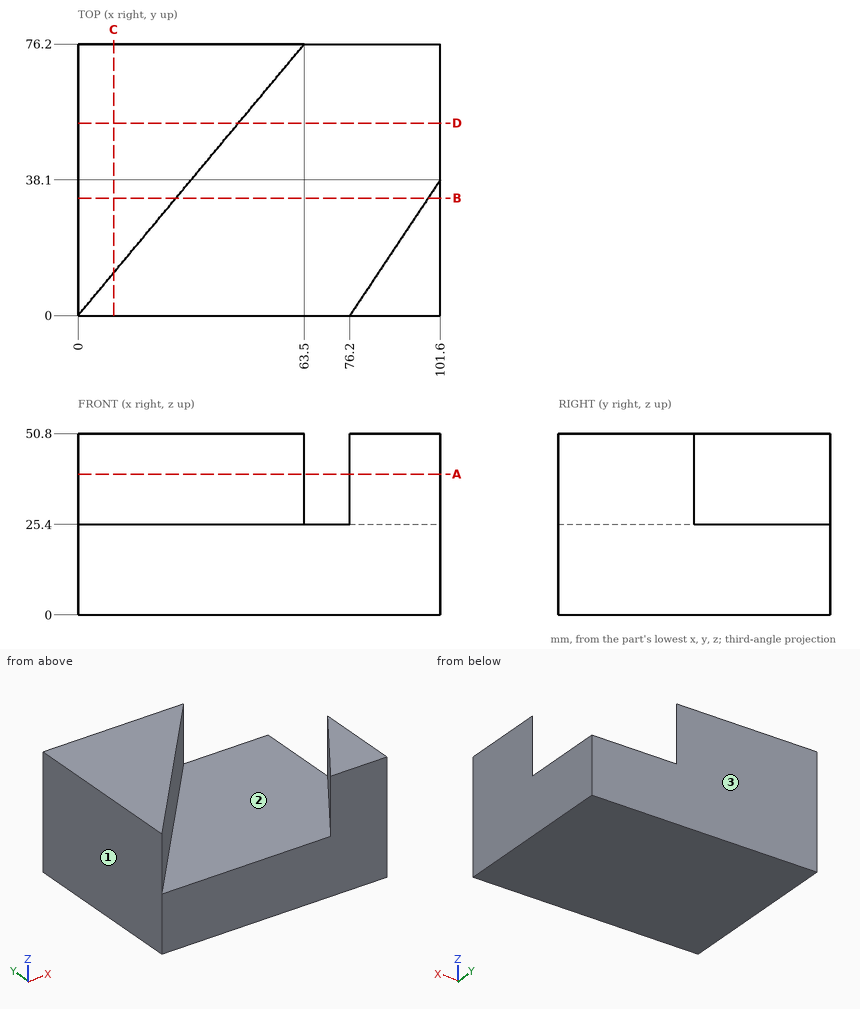
Here's the drawing with two shaded views (mm, measured from the low corner). I have some questions. Round coordinates to 2 decimals unless told otherwise and drop trailing zeros. Write each loop counter-clockwise with the first axis right and the second up, starting at its lowest first coordinate (ties: lowest second). Pieces come first, ordered by that corner, then holes. Notation, with made-up numbers: M 87,-22 L 132,-22 A36 cw 132,13 Z; hole C 16,74.5 d11. An arc over 180 degrees is marked long. Use CSV: the item, a comma, the result in double quotes.
(1) Imagine slicing it at A-A (z = 39.5). Write out the boundary of the cut face in (x, y), plus the area to 3 significant figures.
Check values:
outline,"M 0,0 L 63.5,76.2 L 0,76.2 Z; M 76.2,0 L 101.6,0 L 101.6,38.1 Z"
area,"2,900 mm^2"
(2) I need wall thicknesses on line 1 along Z through (x, y) = (39, 23.5); line 2 along X through (y, z) = (25.5, 26.5); line 3 along X through (y, z) = (18.5, 33.5). Which ranges of each line are inside material? Lowest first, please.
Check values:
line 1,"0 to 25.4"
line 2,"0 to 21.25, 93.2 to 101.6"
line 3,"0 to 15.42, 88.53 to 101.6"
(3) I'm going to push flat-ended pins straight in: pin 1 (10 mm diameter, centred on y = 67.5, z = 45.5, fed in from +X); pin 2 (12 mm diameter, centred on x = 48.5, y = 15.5, fed in from +Z). Where does each tip first touch, or does it pass through?
Check values:
pin 1,"x = 60.42"
pin 2,"z = 25.4"
(4) Imagine slicing it at C-C (x = 10). Write out the boundary of the cut face in (y, z).
Check values:
outline,"M 0,0 L 76.2,0 L 76.2,50.8 L 12,50.8 L 12,25.4 L 0,25.4 Z"
(5) We'd pull the mould along X, two halves only. Please class the marked faces 1, 2 and 3: +X half, -X half, draft (parallel to the pull), parting line (faces both ways), or undercut.
Check values:
face 1,"-X half"
face 2,"undercut"
face 3,"draft"
(6) Imagine slicing it at B-B (y = 33). Write out the boundary of the cut face in (x, z).
Check values:
outline,"M 0,0 L 101.6,0 L 101.6,50.8 L 98.2,50.8 L 98.2,25.4 L 27.5,25.4 L 27.5,50.8 L 0,50.8 Z"
(7) Imagine slicing it at D-D (y = 54). Write out the boundary of the cut face in (x, z), plus the area to 3 significant figures.
Check values:
outline,"M 0,0 L 101.6,0 L 101.6,25.4 L 45,25.4 L 45,50.8 L 0,50.8 Z"
area,"3,720 mm^2"
